The listing builds one solid part. Answer for the finished solid, in the listing's coordinates (mm). Give positions to 0.01 mm unless a question says otherwise; leave off trailing zeros. Order: outer loops, then holes, each group sorted by start corner. A loop starts at its lowest first (then second) coordinate and runs counter-clockwise, first axis right, second up.
Autodesk Inventor part; units mm, degrees
ref_plane "YZ Plane" through (0, 0, 0) normal (1, 0, 0) x (0, 1, 0)
ref_plane "XZ Plane" through (0, 0, 0) normal (0, 1, 0) x (-1, 0, 0)
ref_plane "XY Plane" through (0, 0, 0) normal (0, 0, 1) x (1, 0, 0)
sketch "Esquisse1" plane through (0, 0, 0) normal (0, 1, 0) x (-1, 0, 0)
  line L0 (-75, 50) -> (75, 50)
  line L1 (75, 50) -> (75, -50)
  line L2 (75, -50) -> (-75, -50)
  line L3 (-75, -50) -> (-75, 50)
  line L4 (75, 50) -> (-75, -50) construction
  circle A0 centre (60, -40) radius 1.05
  circle A1 centre (52, -40) radius 1.05
  circle A2 centre (44, -40) radius 1.05
  circle A3 centre (60, -32) radius 1.05
  circle A4 centre (52, -32) radius 1.05 construction
  circle A5 centre (44, -32) radius 1.05
  circle A6 centre (60, -24) radius 1.05
  circle A7 centre (52, -24) radius 1.05
  circle A8 centre (44, -24) radius 1.05
  line L5 (75, 0) -> (-75, 0) construction
  circle A9 centre (60, 40) radius 1.05
  circle A10 centre (52, 40) radius 1.05
  circle A11 centre (44, 40) radius 1.05
  circle A12 centre (60, 32) radius 1.05
  circle A13 centre (52, 32) radius 1.05 construction
  circle A14 centre (44, 32) radius 1.05
  circle A15 centre (60, 24) radius 1.05
  circle A16 centre (52, 24) radius 1.05
  circle A17 centre (44, 24) radius 1.05
  line L6 (64, -2.0284) -> (70, -2.0284)
  line L7 (70, -2.0284) -> (70, -12.0284)
  line L8 (70, -12.0284) -> (64, -12.0284)
  line L9 (64, -12.0284) -> (64, -2.0284)
  line L10 (64, -2.0284) -> (70, -12.0284) construction
  line L11 (70, -2.0284) -> (64, -12.0284) construction
  line L12 (64, 37.9716) -> (70, 37.9716)
  line L13 (70, 37.9716) -> (70, 27.9716)
  line L14 (70, 27.9716) -> (64, 27.9716)
  line L15 (64, 27.9716) -> (64, 37.9716)
  line L16 (64, 37.9716) -> (70, 27.9716) construction
  line L17 (70, 37.9716) -> (64, 27.9716) construction
  line L18 (27, -5.0284) -> (37, -5.0284)
  line L19 (37, -5.0284) -> (37, -11.0284)
  line L20 (37, -11.0284) -> (27, -11.0284)
  line L21 (27, -11.0284) -> (27, -5.0284)
  line L22 (27, -5.0284) -> (37, -11.0284) construction
  line L23 (37, -5.0284) -> (27, -11.0284) construction
  line L24 (27, 36.9716) -> (37, 36.9716)
  line L25 (37, 36.9716) -> (37, 30.9716)
  line L26 (37, 30.9716) -> (27, 30.9716)
  line L27 (27, 30.9716) -> (27, 36.9716)
  line L28 (27, 36.9716) -> (37, 30.9716) construction
  line L29 (37, 36.9716) -> (27, 30.9716) construction
  point P0 (0, 0)
  point P1 (67, -7.0284)
  point P2 (67, 32.9716)
  point P3 (32, -8.0284)
  point P4 (32, 33.9716)
  dimension "d0" = 150
  dimension "d1" = 100
  dimension "d2" = 2.1
  dimension "d3" = 10
  dimension "d4" = 15
  dimension "d7" = 8
  dimension "d10" = 8
  dimension "d25" = 50
  dimension "d26" = 0
  dimension "d27" = 6
  dimension "d28" = 10
  dimension "d29" = 6
  dimension "d30" = 10
  dimension "d31" = 50
  dimension "d32" = 5
  dimension "d33" = 5
  dimension "d34" = 10
  dimension "d35" = 6
  dimension "d36" = 6
  dimension "d37" = 36
  dimension "d38" = 35
  dimension "d39" = 1
ref_plane "Plan de construction1" through (0, 6, 0) normal (0, 1, 0) x (1, 0, 0)
extrude "Extrusion2" add sketch "Esquisse1" along normal blind 6
sketch "Esquisse3" plane through (0, 6, 0) normal (0, 1, 0) x (1, 0, 0)
  line L0 (-37, -36.9716) -> (-37, -30.9716) construction
  line L1 (-37, -30.9716) -> (-27, -30.9716) construction
  line L2 (-27, -30.9716) -> (-27, -36.9716) construction
  line L3 (-27, -36.9716) -> (-37, -36.9716) construction
  line L4 (-37, 5.0284) -> (-37, 11.0284) construction
  line L5 (-37, 11.0284) -> (-27, 11.0284) construction
  line L6 (-27, 11.0284) -> (-27, 5.0284) construction
  line L7 (-27, 5.0284) -> (-37, 5.0284) construction
  line L8 (-70, -37.9716) -> (-70, -27.9716) construction
  line L9 (-70, -27.9716) -> (-64, -27.9716) construction
  line L10 (-64, -27.9716) -> (-64, -37.9716) construction
  line L11 (-64, -37.9716) -> (-70, -37.9716) construction
  line L12 (-70, 2.0284) -> (-70, 12.0284) construction
  line L13 (-70, 12.0284) -> (-64, 12.0284) construction
  line L14 (-64, 12.0284) -> (-64, 2.0284) construction
  line L15 (-64, 2.0284) -> (-70, 2.0284) construction
  circle A0 centre (-60, -40) radius 1.05 construction
  circle A1 centre (-44, -24) radius 1.05 construction
  circle A2 centre (-44, -32) radius 1.05 construction
  circle A3 centre (-44, -40) radius 1.05 construction
  circle A4 centre (-52, -24) radius 1.05 construction
  circle A5 centre (-52, -40) radius 1.05 construction
  circle A6 centre (-60, -24) radius 1.05 construction
  circle A7 centre (-60, -32) radius 1.05 construction
  circle A8 centre (-44, 24) radius 1.05 construction
  circle A9 centre (-52, 24) radius 1.05 construction
  circle A10 centre (-60, 24) radius 1.05 construction
  circle A11 centre (-44, 32) radius 1.05 construction
  circle A12 centre (-60, 32) radius 1.05 construction
  circle A13 centre (-44, 40) radius 1.05 construction
  circle A14 centre (-52, 40) radius 1.05 construction
  circle A15 centre (-60, 40) radius 1.05 construction
  line L16 (-75, -50) -> (75, -50) construction
  line L17 (75, -50) -> (75, 50) construction
  line L18 (75, 50) -> (-75, 50) construction
  line L19 (-75, 50) -> (-75, -50) construction
  line L20 (-27, 8.0284) -> (13, 8.0284) construction
  line L21 (69, -42.5) -> (13, -42.5) construction
  line L22 (13, -42.5) -> (13, 42.5) construction
  line L23 (13, 42.5) -> (69, 42.5) construction
  line L24 (69, 42.5) -> (69, -42.5) construction
  line L25 (69, -42.5) -> (13, 42.5) construction
  line L26 (13, -42.5) -> (69, 42.5) construction
  circle A16 centre (16.75, 38.75) radius 1.5
  circle A17 centre (65.75, 38.75) radius 1.5
  circle A18 centre (16.75, -19.25) radius 1.5
  circle A19 centre (65.75, -19.25) radius 1.5
  point P0 (0, 0)
  point P1 (41, 0)
  dimension "d42" = 40
  dimension "d43" = 56
  dimension "d44" = 85
  dimension "d45" = 0
  dimension "d46" = 3
  dimension "d47" = 3.75
  dimension "d48" = 3.75
  dimension "d51" = 49
  dimension "d54" = 58
extrude "Extrusion3" cut sketch "Esquisse3" against normal blind 6
sketch "Esquisse4" plane through (0, 6, 0) normal (0, 1, 0) x (1, 0, 0)
  line L0 (-40.9885, 18.973) -> (-1.9885, 18.973) construction
  line L1 (-1.9885, 18.973) -> (-1.9885, 43.973) construction
  line L2 (-1.9885, 43.973) -> (-40.9885, 43.973) construction
  line L3 (-40.9885, 43.973) -> (-40.9885, 18.973) construction
  line L4 (-40.9885, 18.973) -> (-1.9885, 43.973) construction
  line L5 (-1.9885, 18.973) -> (-40.9885, 43.973) construction
  circle A0 centre (-40.9885, 43.973) radius 2
  circle A1 centre (-40.9885, 18.973) radius 2
  point P0 (0, 0)
  point P1 (-21.4885, 31.473)
  dimension "d59" = 39
  dimension "d60" = 25
  dimension "d61" = 4
  dimension "d62" = 4
extrude "Extrusion4" cut sketch "Esquisse4" against normal blind 10
sketch "Esquisse5" plane through (0, 6, 0) normal (0, 1, 0) x (1, 0, 0)
  line L0 (9, -3) -> (19, -3)
  line L1 (19, -3) -> (19, 3)
  line L2 (19, 3) -> (9, 3)
  line L3 (9, 3) -> (9, -3)
  line L4 (9, -3) -> (19, 3) construction
  line L5 (19, -3) -> (9, 3) construction
  line L6 (59, -3) -> (69, -3)
  line L7 (69, -3) -> (69, 3)
  line L8 (69, 3) -> (59, 3)
  line L9 (59, 3) -> (59, -3)
  line L10 (59, -3) -> (69, 3) construction
  line L11 (69, -3) -> (59, 3) construction
  line L12 (75, 50) -> (75, -50)
  point P0 (0, 0)
  point P1 (14, 0)
  point P2 (64, 0)
  dimension "d65" = 10
  dimension "d66" = 6
  dimension "d67" = 10
  dimension "d68" = 6
  dimension "d71" = 60
  dimension "d72" = 6
extrude "Extrusion5" cut sketch "Esquisse5" against normal blind 10
properties part number "base"
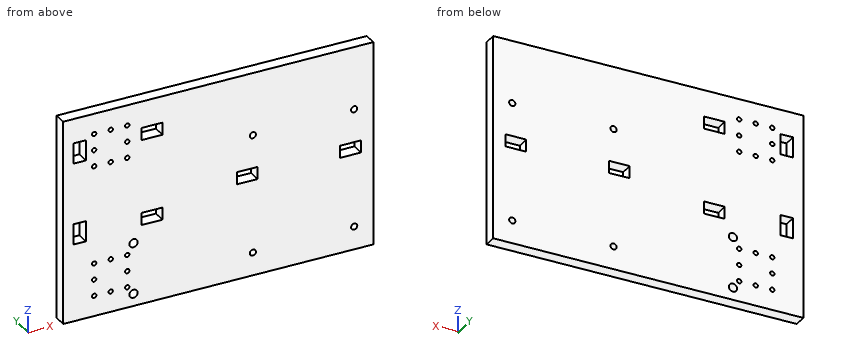
1) Find section C-C (z = -8). Write down the section's boundary in (x, y).
Geometry says:
outline: (-75, 0) - (-70, 0) - (-70, 6) - (-75, 6) - close; (-64, 0) - (-37, 0) - (-37, 6) - (-64, 6) - close; (-27, 0) - (75, 0) - (75, 6) - (-27, 6) - close
2) Find section D-D (y = 3.6). Count the separate pieces of the cut face and the enclosed holes in it, then the cut area to 3 significant figures.
Geometry says:
separate pieces: 1
enclosed holes: 28
area: 14,500 mm2
3) Straight lines are drawn through the part: probe 1 along X at (y, z) = (0.6, 2); probe 2 along Z at (x, y) = (65.75, 1.3); probe 3 along X at (y, z) = (3.85, -7.5). For each, find the intervals that lie inside material, in ascending order.
Geometry says:
probe 1: x = -75 to 9, 19 to 59, 69 to 75
probe 2: z = -50 to -40.25, -37.25 to -3, 3 to 17.75, 20.75 to 50
probe 3: x = -75 to -70, -64 to -37, -27 to 75
4) Find section A-A (z = 19.25). Write down the section's boundary in (x, y), then the cut area to 3 significant figures.
Geometry says:
outline: (-75, 0) - (15.25, 0) - (15.25, 6) - (-75, 6) - close; (18.25, 0) - (64.25, 0) - (64.25, 6) - (18.25, 6) - close; (67.25, 0) - (75, 0) - (75, 6) - (67.25, 6) - close
area: 864 mm2
5) Find section B-B (x = 65.75). Write down the section's boundary in (y, z).
Geometry says:
outline: (0, -50) - (6, -50) - (6, -40.25) - (0, -40.25) - close; (0, -37.25) - (6, -37.25) - (6, -3) - (0, -3) - close; (0, 3) - (6, 3) - (6, 17.75) - (0, 17.75) - close; (0, 20.75) - (6, 20.75) - (6, 50) - (0, 50) - close
